Read the model definition and answer for the solid it produces. Units are mm, in the model's axes. Round coordinates to 2 decimals unless told otherwise and drop trailing zeros. Write each loop counter-clockwise with the first axis right and the second up, starting at its lowest first coordinate (ties: lowest second). Pieces come first, ordered by that corner, then holes.
Autodesk Inventor part; units mm, degrees
ref_plane "YZ Plane" through (0, 0, 0) normal (1, 0, 0) x (0, 1, 0)
ref_plane "XZ Plane" through (0, 0, 0) normal (0, 1, 0) x (-1, 0, 0)
ref_plane "XY Plane" through (0, 0, 0) normal (0, 0, 1) x (1, 0, 0)
sketch "스케치1" plane through (0, 0, 0) normal (0, 0, 1) x (1, 0, 0)
  line L0 (0, 0) -> (-24, 0)
  line L1 (-24, 0) -> (-24, 38)
  line L2 (-20, 42) -> (-4, 42)
  line L3 (0, 38) -> (0, 0)
  arc A0 (0, 38) -> (-4, 42) centre (-4, 38) ccw
  arc A1 (-20, 42) -> (-24, 38) centre (-20, 38) ccw
  circle A2 centre (-12, 27) radius 7.55
  point P0 (-24, 42)
  point P1 (0, 42)
  dimension "d0" = 24
  dimension "d1" = 42
  dimension "d2" = 4
  dimension "d4" = 15.1
extrude "돌출1" add sketch "스케치1" along normal blind 5
properties part number "베어링받침대" material "알루미늄 6061"
Q1. Section B-B (x = -12) is taken. Determine the outline of the cut face in (y, z).
Verdict:
outline: (0, 0) - (19.45, 0) - (19.45, 5) - (0, 5) - close; (34.55, 0) - (42, 0) - (42, 5) - (34.55, 5) - close
Q2. Determine the mould class of faces 1 (the flat face through (-24, 19, 2)), 2 (the cylindrical face through (-12.983, 19.514, 2.465)), 3 (the cylindrical face through (-1.203, 40.859, 2.465)), 4 (the flat face through (-12, 42, 2)) for opening direction X: pulls with the +X half, pulls with the -X half, needs draft (parallel to the pull), parting line crosses it, or undercut.
Verdict:
face 1: pulls with the -X half
face 2: undercut
face 3: pulls with the +X half
face 4: needs draft
Q3. A flat-ended cylindrical pin translates along its axis: pin 1 Ø9 at (x, y) = (-12, 27) entering from -Z. Find the tip coordinate at first contact, or state that the pin passes through.
Verdict:
pin 1: passes through
Q4. Straight lines are drawn through the part: probe 1 along Y at (x, z) = (-12, 2.8); probe 2 along Y at (x, z) = (-8.5, 1.5); probe 3 along X at (y, z) = (30, 2.25). For each, find the intervals that lie inside material, in ascending order.
Verdict:
probe 1: y = 0 to 19.45, 34.55 to 42
probe 2: y = 0 to 20.31, 33.69 to 42
probe 3: x = -24 to -18.93, -5.07 to 0
Q5. Section A-A (y = 27) is taken. Determine the outline of the cut face in (x, z), then the cut area to 3 significant figures.
Verdict:
outline: (-24, 0) - (-19.55, 0) - (-19.55, 5) - (-24, 5) - close; (-4.45, 0) - (0, 0) - (0, 5) - (-4.45, 5) - close
area: 44.5 mm2
Q6. Section C-C (z = 1.85) is taken. Determine the outline of the cut face in (x, y), then the cut area to 3 significant figures.
Verdict:
outline: (-24, 0) - (0, 0) - (0, 38) arc R4 ccw to (-4, 42) - (-20, 42) arc R4 ccw to (-24, 38) - close; hole circle Ø15.1 at (-12, 27)
area: 822 mm2
